Could you check a few things on this model? Use its own coordinates, in mm. Face numbers are marked on the shaded views. A direction names the side the tool comes from. Coordinates: 2 decimals unless noted, no trailing zeros. Loops run counter-clockwise (first coordinate to the right, second up) from the corner with the lowest first, then second, coordinate; pieces in that order, holes last.
from build123d import *

# Parameters (mm, degrees)
F1_DEPTH = 10
F2_W     = 130
F2_H     = 80
F2_W_2   = 110
F2_H_2   = 60
F3_DEPTH = 60
F4_W     = 20
F4_H     = 10
F4_W_2   = 10
F4_H_2   = 20
F5_DEPTH = 10
F6_R     = 5
F8_DEPTH = 25
F9_R     = 7.49999


# Not quite as in the source:
# - a fillet or chamfer is up to 0.001 mm smaller than in the source, because OpenCascade refuses the exact size


with BuildPart() as f1:
    # F0 (on Top) → F1 (new body)
    with BuildSketch(Plane.XY):
        Polygon((55, 40), (-55, 40), (-65, 40), (-65, -40), (-55, -40), (65, -40), (65, -30), (65, 40), align=None)
    extrude(amount=F1_DEPTH)

    # F2 (on face) → F3 (join)
    with BuildSketch(Plane.XY.offset(10)):
        Rectangle(F2_W, F2_H)
        Rectangle(F2_W_2, F2_H_2, mode=Mode.SUBTRACT)
    extrude(amount=F3_DEPTH)

    # F4 (on face) → F5 (cut)
    with BuildSketch(Plane.XY.offset(70)):
        Polygon((10, 30), (10, 40), (0, 40), (-10, 40), (-10, 30), align=None)
        Polygon((-65, 0), (-65, -10), (-55, -10), (-55, 10), (-65, 10), align=None)
        with Locations((0, -35)):
            Rectangle(F4_W, F4_H)
        with Locations((60, 0)):
            Rectangle(F4_W_2, F4_H_2)
    extrude(amount=-F5_DEPTH, mode=Mode.SUBTRACT)

    # F6
    f6_edges = [f1.edges().sort_by_distance(p)[0] for p in [
        (-65, -40, 35),
        (65, -40, 35),
        (-65, 40, 35),
        (65, 40, 35),
    ]]
    fillet(f6_edges, radius=F6_R)

    # F7 (on face) → F8 (cut)
    with BuildSketch(Plane.YZ.offset(65)):
        Polygon((-25, 10), (0, 10), (25, 10), (25, 25), (-25, 25), align=None)
    extrude(amount=-F8_DEPTH, mode=Mode.SUBTRACT)

    # F9 (radius 7.5 in the source; OpenCascade refuses exactly that, so slightly less here)
    f9_edges = [f1.edges().sort_by_distance(p)[0] for p in [
        (60, 25, 25),
        (60, 25, 10),
        (60, -25, 10),
        (60, -25, 25),
    ]]
    fillet(f9_edges, radius=F9_R)


solid = f1.part
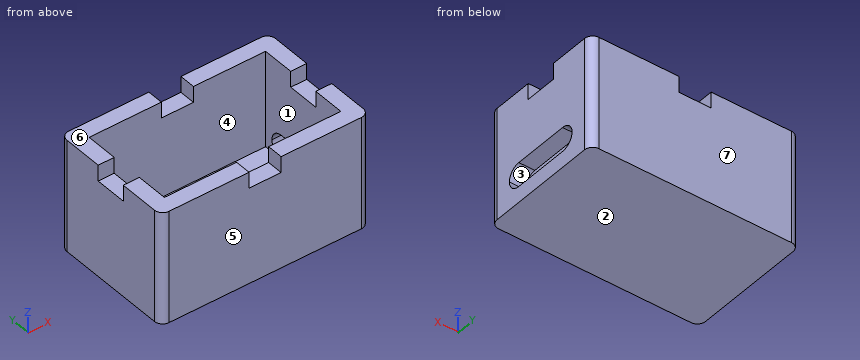
(1) Which directions (+Z, -Z, +X, -X, +Y, -Y) give clear straight access to the entire face, cutting with the end or side of a thin tool? Please do the marked faces 1, 2 and 3.
Answers:
face 1: +Z
face 2: -Z, +X, -X, +Y, -Y
face 3: +X
(2) Imagine slicing it at C-C, the plane z = 30.5. Write out the boundary of the cut face in (x, y).
Answers:
outline: (-65, -35) arc R5 ccw to (-60, -40) - (60, -40) arc R5 ccw to (65, -35) - (65, 35) arc R5 ccw to (60, 40) - (-60, 40) arc R5 ccw to (-65, 35) - close; hole (-55, -30) - (55, -30) - (55, 30) - (-55, 30) - close
(3) Imagine slicing it at A-A, the plane y = 0. Write out the boundary of the cut face in (x, z), and give its area (3 significant figures).
Answers:
outline: (-65, 0) - (65, 0) - (65, 10) - (-55, 10) - (-55, 60) - (-65, 60) - close; (55, 25) - (65, 25) - (65, 60) - (55, 60) - close
area: 2,150 mm2
(4) Imagine slicing it at D-D, the plane z = 11.5. Write out the boundary of the cut face in (x, y).
Answers:
outline: (-65, -35) arc R5 ccw to (-60, -40) - (60, -40) arc R5 ccw to (65, -35) - (65, -22) - (55, -22) - (55, -30) - (-55, -30) - (-55, 30) - (55, 30) - (55, 22) - (65, 22) - (65, 35) arc R5 ccw to (60, 40) - (-60, 40) arc R5 ccw to (-65, 35) - close
(5) For pin 1 (3 mm diameter, centred on x = -61, z = 63, fed in from -Y); pin 2 (8 mm diameter, centred on x = 61, y = 4, fed in from +Z); pin 3 (3 mm diameter, centred on y = 37, z = 63.5, fed in from -X), each with a flat end and sliding along its axis, tell me the tip position at first contact or that it passes through.
Answers:
pin 1: stops at y = -40
pin 2: stops at z = 60
pin 3: stops at x = -64.97
(6) Imagine slicing it at B-B, the plane x = 5. Write out the boundary of the cut face in (y, z).
Answers:
outline: (-40, 0) - (40, 0) - (40, 60) - (30, 60) - (30, 10) - (-30, 10) - (-30, 60) - (-40, 60) - close
(7) I need wall thicknesses on probe 1 along Y at (x, z) = (-6, 37.5); probe 2 along X at (y, z) = (26.5, 29); probe 3 along Z at (x, y) = (-40.5, -2.5). Which ranges of each line are inside material? Lowest first, please.
Answers:
probe 1: y = -40 to -30, 30 to 40
probe 2: x = -65 to -55, 55 to 65
probe 3: z = 0 to 10
(8) We'd pull the mould along Y, two halves only. Please class the marked faces 4, 5, 6 and 7: +Y half, -Y half, draft (parallel to the pull), parting line (faces both ways), or undercut.
Answers:
face 4: undercut
face 5: -Y half
face 6: draft
face 7: +Y half
